Autodesk Inventor part; units mm, degrees
ref_plane "YZ Plane" through (0, 0, 0) normal (1, 0, 0) x (0, 1, 0)
ref_plane "XZ Plane" through (0, 0, 0) normal (0, 1, 0) x (-1, 0, 0)
ref_plane "XY Plane" through (0, 0, 0) normal (0, 0, 1) x (1, 0, 0)
sketch "Náčrt1" plane through (0, 0, 0) normal (1, 0, 0) x (0, 1, 0)
  line L0 (0, 0) -> (80, 0)
  line L1 (80, 0) -> (80, -6)
  line L2 (80, -6) -> (6, -6)
  line L3 (6, -6) -> (6, -154)
  line L4 (6, -154) -> (80, -154)
  line L5 (80, -154) -> (80, -160)
  line L6 (80, -160) -> (0, -160)
  line L7 (0, -160) -> (0, 0)
  dimension "d0" = 80
  dimension "d1" = 6
  dimension "d3" = 148
  dimension "d5" = 6
  dimension "d6" = 80
  dimension "d20" = 160
  dimension "d21" = 74
extrude "Vysunutí1" add sketch "Náčrt1" along normal blind 380
sketch "Náčrt4" plane through (0, 6, -6) normal (0, 1, 0) x (1, 0, 0)
  line L0 (0, 0) -> (0, 148)
  line L1 (0, 0) -> (380, 0)
  line L2 (380, 148) -> (380, 0)
  line L3 (0, 148) -> (380, 148)
  circle A0 centre (355, 74) radius 5.25
  line L4 (0, 154) -> (380, 154)
  point P0 (0, -6)
  dimension "d14" = 25
  dimension "d15" = 80
  dimension "d16" = 10.5
extrude "Vysunutí3" cut sketch "Náčrt4" against normal through all contours A0
sketch "Náčrt5" plane through (0, 0, 0) normal (0, 0, 1) x (1, 0, 0)
  circle A0 centre (23, 46) radius 5.25
  line L0 (380, 80) -> (380, 0)
  line L1 (0, 0) -> (380, 0)
  dimension "d22" = 10.5
  dimension "d23" = 357
  dimension "d24" = 46
extrude "Vysunutí4" cut sketch "Náčrt5" against normal through all
sketch "Náčrt6" plane through (0, 0, -160) normal (0, 0, -1) x (-1, 0, 0)
  circle A0 centre (-23, 46) radius 5.25
  line L0 (0, 80) -> (0, 0)
  line L1 (0, 80) -> (-380, 80)
  line L2 (-380, 0) -> (-380, 80)
  line L3 (0, 0) -> (-380, 0)
  line L4 (-219.2388, 40) -> (-154.125, 40)
  line L5 (-190, 7.0383) -> (-190, 75.4408)
  arc A1 (-216.8837, 45.7895) -> (-209.5518, 44.2105) centre (-213.2177, 45) ccw
  arc A2 (-209.5518, 35.7895) -> (-216.8837, 34.2105) centre (-213.2177, 35) ccw
  arc A3 (-195.7895, 13.1163) -> (-194.2105, 20.4482) centre (-195, 16.7823) ccw
  arc A4 (-185.7895, 20.4482) -> (-184.2105, 13.1163) centre (-185, 16.7823) ccw
  arc A5 (-163.1163, 34.2105) -> (-170.4482, 35.7895) centre (-166.7823, 35) ccw
  arc A6 (-170.4482, 44.2105) -> (-163.1163, 45.7895) centre (-166.7823, 45) ccw
  arc A7 (-184.2105, 66.8837) -> (-185.7895, 59.5518) centre (-185, 63.2177) ccw
  arc A8 (-194.2105, 59.5518) -> (-195.7895, 66.8837) centre (-195, 63.2177) ccw
  arc A9 (-194.2105, 59.5518) -> (-209.5518, 44.2105) centre (-190, 40) ccw
  arc A10 (-195.7895, 66.8837) -> (-216.8837, 45.7895) centre (-190, 40) ccw
  arc A11 (-163.1163, 45.7895) -> (-184.2105, 66.8837) centre (-190, 40) ccw
  arc A12 (-170.4482, 44.2105) -> (-185.7895, 59.5518) centre (-190, 40) ccw
  arc A13 (-216.8837, 34.2105) -> (-195.7895, 13.1163) centre (-190, 40) ccw
  arc A14 (-184.2105, 13.1163) -> (-163.1163, 34.2105) centre (-190, 40) ccw
  arc A15 (-209.5518, 35.7895) -> (-194.2105, 20.4482) centre (-190, 40) ccw
  arc A16 (-185.7895, 20.4482) -> (-170.4482, 35.7895) centre (-190, 40) ccw
  point P0 (0, 0)
  dimension "d22" = 10.5
  dimension "d29" = 190
  dimension "d30" = 40
  dimension "d31" = 5
  dimension "d32" = 5
  dimension "d35" = 360
extrude "Vysunutí5" cut sketch "Náčrt6" against normal up to surface (6 mm away) contours A10 A8 A9 A1 | A15 A3 A13 A2 | A16 A5 A14 A4 | A12 A7 A11 A6
properties part number "U profil"
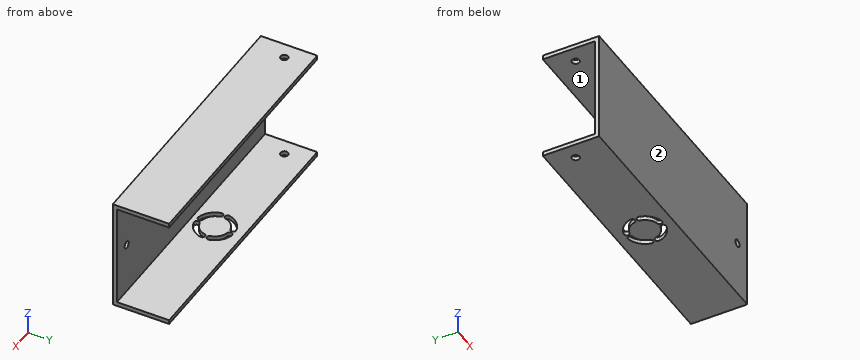
Input: part model. Units: mm. Frame: model coordinates. Face numbers are marked on the shaded views. A direction names the side the tool comes from. Round coordinates to 2 decimals unless told otherwise and drop trailing zeros. Write each loop counter-clockwise with the first axis right and the second up, starting at its lowest first coordinate (ties: lowest second). Pieces come first, ordered by that corner, then holes.
1) Ray query, L1, parallel to Z at x = 31.5, y = 70; L2, parallel to X at y = 1, z = -80; L3, parallel to Y at x = 23, z = -4. Return the intervals inside material, ascending.
2) Cut plane D-D (x = 355). Return the cut outline in (y, z), then the cut area to 4 significant figures.
3) Cut plane A-A (x = 23). Return the cut outline in (y, z), then the cut area to 3 significant figures.
4) Reachability of the marked faces 1 and 2 from +Z, -Z, +X, -X, +Y, -Y: full face, straight path, thin tool, end or side. Return the list, or none.
5) Cut plane C-C (y = 27.5). Return the cut outline in (x, z), then the cut area to 3 significant figures.
6) Cut plane B-B (z = -80). Return the cut outline in (x, y), then the cut area to 3 significant figures.
Geometry says:
1. L1: z = -160 to -154, -6 to 0
1. L2: x = 0 to 349.75, 360.25 to 380
1. L3: y = 0 to 40.75, 51.25 to 80
2. outline: (0, -160) - (80, -160) - (80, -154) - (6, -154) - (6, -85.25) - (0, -85.25) - close; (0, -74.75) - (6, -74.75) - (6, -6) - (80, -6) - (80, 0) - (0, 0) - close
2. area: 1,785 mm2
3. outline: (0, -160) - (40.75, -160) - (40.75, -154) - (6, -154) - (6, -6) - (40.75, -6) - (40.75, 0) - (0, 0) - close; (51.25, -160) - (80, -160) - (80, -154) - (51.25, -154) - close; (51.25, -6) - (80, -6) - (80, 0) - (51.25, 0) - close
3. area: 1,720 mm2
4. face 1: +X, -X, +Y
4. face 2: +Z, -Z, +X, -X, -Y
5. outline: (0, -160) - (165.51, -160) - (165.51, -154) - (0, -154) - close; (0, -6) - (380, -6) - (380, 0) - (0, 0) - close; (174.39, -160) - (205.61, -160) - (205.61, -154) - (174.39, -154) - close; (214.49, -160) - (380, -160) - (380, -154) - (214.49, -154) - close
5. area: 4,450 mm2
6. outline: (0, 0) - (349.75, 0) - (349.75, 6) - (0, 6) - close; (360.25, 0) - (380, 0) - (380, 6) - (360.25, 6) - close
6. area: 2,220 mm2
